```python
from build123d import *

# Parameters (mm, degrees)
BOSS_EXTRUDE1_DEPTH     = 10
SKETCH2_W               = 17.2
SKETCH2_H               = 43
CUT_EXTRUDE1_DEPTH      = 72.414284285
SKETCH3_W               = 90
SKETCH3_H               = 34
SKETCH3_W_2             = 80
SKETCH3_H_2             = 24
BOSS_EXTRUDE3_DEPTH     = 15
SKETCH4_W               = 49.6
SKETCH4_H               = 5
BOSS_EXTRUDE4_DEPTH     = 10
SKETCH5_W               = 15
SKETCH5_H               = 22
BOSS_EXTRUDE5_DEPTH     = 5
SKETCH6_W               = 90
SKETCH6_H               = 77
BOSS_EXTRUDE6_DEPTH     = 15
BOSS_EXTRUDE8_DEPTH     = 39
CHAMFER1_SIZE           = 64
CHAMFER1_SIZE_2         = 3.354097874
CHAMFER2_SIZE           = 64
CHAMFER2_SIZE_2         = 11.405813635
CHAMFER3_SIZE           = 64
CHAMFER3_SIZE_2         = 13.775745352
CUT_EXTRUDE3_DEPTH      = 95.500525601
CUT_EXTRUDE3_DEPTH_BACK = 95.500525601
SKETCH10_W              = 50
SKETCH10_H              = 27
SKETCH15_R              = 8
CUT_EXTRUDE5_DEPTH      = 122.227059686
CUT_EXTRUDE6_DEPTH      = 2.5
SKETCH18_W              = 29.6
SKETCH18_H              = 43
CUT_EXTRUDE7_DEPTH      = 10
CUT_EXTRUDE8_DEPTH      = 15
SKETCH21_W              = 29.6
SKETCH21_H              = 33
BOSS_EXTRUDE10_DEPTH    = 2.5
SKETCH23_W              = 2.05
SKETCH23_H              = 13
BOSS_EXTRUDE11_DEPTH    = 15
SKETCH24_W              = 90
SKETCH24_H              = 72
CUT_EXTRUDE9_DEPTH      = 54


with BuildPart() as part:
    # Sketch1 → Boss-Extrude1 (new body)
    with BuildSketch(Plane(origin=(0, 0, 0), x_dir=(1, 0, 0), z_dir=(0, 1, 0))):
        with BuildLine():
            Line((-35, 50), (35, 50))
            ThreePointArc((35, 50), (45.606601718, 45.606601718), (50, 35))
            Line((50, 35), (50, -35))
            ThreePointArc((50, -35), (45.606601718, -45.606601718), (35, -50))
            Line((35, -50), (-35, -50))
            ThreePointArc((-35, -50), (-45.606601718, -45.606601718), (-50, -35))
            Line((-50, -35), (-50, 35))
            ThreePointArc((-50, 35), (-45.606601718, 45.606601718), (-35, 50))
        make_face()
    extrude(amount=BOSS_EXTRUDE1_DEPTH)

    # Sketch2 → Cut-Extrude1 (cut, through all)
    with BuildSketch(Plane(origin=(0, 10, 0), x_dir=(1, 0, 0), z_dir=(0, 1, 0))):
        with Locations((-33.4, 18.5)):
            Rectangle(SKETCH2_W, SKETCH2_H)
        with Locations((33.4, 18.5)):
            Rectangle(SKETCH2_W, SKETCH2_H)
    extrude(amount=-CUT_EXTRUDE1_DEPTH, mode=Mode.SUBTRACT)

    # Sketch3 → Boss-Extrude3 (add)
    with BuildSketch(Plane(origin=(0, 10, 0), x_dir=(1, 0, 0), z_dir=(0, 1, 0))):
        with Locations((0, -20)):
            Rectangle(SKETCH3_W, SKETCH3_H)
        with Locations((0, -20)):
            Rectangle(SKETCH3_W_2, SKETCH3_H_2, mode=Mode.SUBTRACT)
    extrude(amount=BOSS_EXTRUDE3_DEPTH)

    # Sketch4 → Boss-Extrude4 (add)
    with BuildSketch(Plane(origin=(0, 10, 0), x_dir=(1, 0, 0), z_dir=(0, 1, 0))):
        with Locations((0, 10)):
            Rectangle(SKETCH4_W, SKETCH4_H)
        with Locations((0, 27)):
            Rectangle(SKETCH4_W, SKETCH4_H)
    extrude(amount=BOSS_EXTRUDE4_DEPTH)

    # Sketch5 → Boss-Extrude5 (add)
    with BuildSketch(Plane(origin=(0, 20, 0), x_dir=(1, 0, 0), z_dir=(0, 1, 0))):
        with Locations((-17.3, 18.5)):
            Rectangle(SKETCH5_W, SKETCH5_H)
        with Locations((17.3, 18.5)):
            Rectangle(SKETCH5_W, SKETCH5_H)
    extrude(amount=BOSS_EXTRUDE5_DEPTH)

    # Sketch6 → Boss-Extrude6 (add)
    with BuildSketch(Plane(origin=(0, 10, 0), x_dir=(1, 0, 0), z_dir=(0, 1, 0))):
        with BuildLine():
            Line((-50, 35), (-50, -35))
            ThreePointArc((-50, -35), (-45.606601718, -45.606601718), (-35, -50))
            Line((-35, -50), (35, -50))
            ThreePointArc((35, -50), (45.606601718, -45.606601718), (50, -35))
            Line((50, -35), (50, 35))
            ThreePointArc((50, 35), (45.606601718, 45.606601718), (35, 50))
            Line((35, 50), (-35, 50))
            ThreePointArc((-35, 50), (-45.606601718, 45.606601718), (-50, 35))
        make_face()
        with Locations((0, 1.5)):
            Rectangle(SKETCH6_W, SKETCH6_H, mode=Mode.SUBTRACT)
    extrude(amount=BOSS_EXTRUDE6_DEPTH)

    # Sketch9 → Boss-Extrude8 (add)
    with BuildSketch(Plane(origin=(0, 25, 0), x_dir=(1, 0, 0), z_dir=(0, 1, 0))):
        with BuildLine():
            Line((-50, 35), (-50, -35))
            ThreePointArc((-50, -35), (-45.606601718, -45.606601718), (-35, -50))
            Line((-35, -50), (35, -50))
            ThreePointArc((35, -50), (45.606601718, -45.606601718), (50, -35))
            Line((50, -35), (50, 35))
            ThreePointArc((50, 35), (45.606601718, 45.606601718), (35, 50))
            Line((35, 50), (-35, 50))
            ThreePointArc((-35, 50), (-45.606601718, 45.606601718), (-50, 35))
        make_face()
        with BuildLine():
            Line((-45, 35), (-45, -32))
            Line((-45, -32), (45, -32))
            Line((45, -32), (45, 35))
            ThreePointArc((45, 35), (44.659258263, 37.588190451), (43.660254038, 40))
            Line((43.660254038, 40), (-43.660254038, 40))
            ThreePointArc((-43.660254038, 40), (-44.659258263, 37.588190451), (-45, 35))
        make_face(mode=Mode.SUBTRACT)
    extrude(amount=BOSS_EXTRUDE8_DEPTH)

    # Chamfer1
    # the kernel refuses this chamfer: 64, 3.354097874 mm, written as the material it takes off along each edge
    with BuildSketch(Plane(origin=(-35, 64, 50), x_dir=(0, -0.9999979738662979, 0.002013023422382214), z_dir=(1, 0, 0)), Plane(origin=(50, 64, 35), x_dir=(0.002013023422382214, -0.9999979738662979, 0), z_dir=(0, 0, -1)), Plane(origin=(-50, 64, -35), x_dir=(-0.002013023422382214, -0.9999979738662979, 0), z_dir=(0, 0, 1)), Plane(origin=(35, 64, -50), x_dir=(0, -0.9999979738662979, -0.002013023422382214), z_dir=(-1, 0, 0))) as chamfer1_piece_1:
        Polygon((CHAMFER1_SIZE * 0.999997973866, CHAMFER1_SIZE * 0.00201302342238), (-CHAMFER1_SIZE_2 * 0.00201302342245, CHAMFER1_SIZE_2 * 0.9999979739), (0, 0), align=None)
    extrude(amount=70, mode=Mode.SUBTRACT)
    with BuildSketch(Plane(origin=(35, 64, 35), x_dir=(0, 0, 1), z_dir=(-1, 0, 0))) as chamfer1_piece_2:
        Polygon((15, -CHAMFER1_SIZE), (15 - CHAMFER1_SIZE_2, 0), (15, 0), align=None)
    revolve(axis=Axis((35, 64, 35), (0, 1, 0)), revolution_arc=90, mode=Mode.SUBTRACT)
    with BuildSketch(Plane(origin=(-35, 64, 35), x_dir=(-1, 0, 0), z_dir=(0, 0, -1))) as chamfer1_piece_3:
        Polygon((15, -CHAMFER1_SIZE), (15 - CHAMFER1_SIZE_2, 0), (15, 0), align=None)
    revolve(axis=Axis((-35, 64, 35), (0, 1, 0)), revolution_arc=90, mode=Mode.SUBTRACT)
    with BuildSketch(Plane(origin=(35, 64, -35), x_dir=(1, 0, 0), z_dir=(0, 0, 1))) as chamfer1_piece_4:
        Polygon((15, -CHAMFER1_SIZE), (15 - CHAMFER1_SIZE_2, 0), (15, 0), align=None)
    revolve(axis=Axis((35, 64, -35), (0, 1, 0)), revolution_arc=90, mode=Mode.SUBTRACT)
    with BuildSketch(Plane(origin=(-35, 64, -35), x_dir=(0, 0, -1), z_dir=(1, 0, 0))) as chamfer1_piece_5:
        Polygon((15 - CHAMFER1_SIZE_2, 0), (15, -CHAMFER1_SIZE), (15, 0), align=None)
    revolve(axis=Axis((-35, 64, -35), (0, 1, 0)), revolution_arc=90, mode=Mode.SUBTRACT)

    # Chamfer2
    # the kernel refuses this chamfer: 64, 11.405813635 mm, written as the material it takes off along each edge
    with BuildSketch(Plane(origin=(201.306482971, 64, -46.645902126), x_dir=(0, -0.9982575003065525, -0.05900816114499234), z_dir=(-1, 0, 0))) as chamfer2_piece_1:
        Polygon((CHAMFER2_SIZE * 0.999977671636, CHAMFER2_SIZE * 0.0066825316561), (-CHAMFER2_SIZE_2 * 0.0590081611462, CHAMFER2_SIZE_2 * 0.998257500326), (0, 0), align=None)
    extrude(amount=402.612965942, mode=Mode.SUBTRACT)

    # Chamfer3
    # the kernel refuses this chamfer: 64, 13.775745352 mm, written as the material it takes off along each edge
    with BuildSketch(Plane(origin=(-201.265469314, 64, 46.645902126), x_dir=(0, -0.9981787050157903, 0.06032638604292662), z_dir=(1, 0, 0))) as chamfer3_piece_1:
        Polygon((CHAMFER3_SIZE * 0.999967974892, CHAMFER3_SIZE * 0.00800307379952), (-CHAMFER3_SIZE_2 * 0.060326386045, CHAMFER3_SIZE_2 * 0.99817870505), (0, 0), align=None)
    extrude(amount=402.530938629, mode=Mode.SUBTRACT)

    # Sketch10 → Cut-Extrude3 (cut, two sides: drawn at the far end of the back side and taken through both)
    with BuildSketch(Plane(origin=(0, 1.307501734, 0), x_dir=(0, 0, 1), z_dir=(-1, 0, 0)).offset(-CUT_EXTRUDE3_DEPTH_BACK)):
        with Locations((-22.129843227, 49.192498266)):
            Rectangle(SKETCH10_W, SKETCH10_H)
    extrude(amount=CUT_EXTRUDE3_DEPTH + CUT_EXTRUDE3_DEPTH_BACK, mode=Mode.SUBTRACT)

    # Sketch15 → Cut-Extrude5 (cut, through all)
    with BuildSketch(Plane.XY.offset(-40)):
        with Locations((-12.75, 20.25)):
            Circle(SKETCH15_R)
        with Locations((12.75, 20.25)):
            Circle(SKETCH15_R)
    extrude(amount=-CUT_EXTRUDE5_DEPTH, mode=Mode.SUBTRACT)

    # Sketch17 → Cut-Extrude6 (cut)
    with BuildSketch(Plane(origin=(0, 0, -29.5), x_dir=(-1, 0, 0), z_dir=(0, 0, -1))):
        Polygon((-24.8, 10), (24.8, 10), (24.8, 25), (9.8, 25), (9.8, 20), (-9.8, 20), (-9.8, 25), (-24.8, 25), align=None)
    extrude(amount=-CUT_EXTRUDE6_DEPTH, mode=Mode.SUBTRACT)

    # Sketch18 → Cut-Extrude7 (cut)
    with BuildSketch(Plane.XZ):
        with Locations((0, -18.5)):
            Rectangle(SKETCH18_W, SKETCH18_H)
    extrude(amount=-CUT_EXTRUDE7_DEPTH, mode=Mode.SUBTRACT)

    # Sketch20 → Cut-Extrude8 (cut)
    with BuildSketch(Plane.XZ.offset(-25)):
        with BuildLine():
            Line((-45, -35), (-45, -40))
            Line((-45, -40), (-43.660254038, -40))
            ThreePointArc((-43.660254038, -40), (-44.659258263, -37.588190451), (-45, -35))
        make_face()
        with BuildLine():
            Line((45, -40), (45, -35))
            ThreePointArc((45, -35), (44.659258263, -37.588190451), (43.660254038, -40))
            Line((43.660254038, -40), (45, -40))
        make_face()
    extrude(amount=-CUT_EXTRUDE8_DEPTH, mode=Mode.SUBTRACT)

    # Sketch21 → Boss-Extrude10 (add)
    with BuildSketch(Plane.XZ):
        with Locations((0, -13.5)):
            Rectangle(SKETCH21_W, SKETCH21_H)
    extrude(amount=-BOSS_EXTRUDE10_DEPTH)

    # Sketch23 → Boss-Extrude11 (add)
    with BuildSketch(Plane(origin=(0, 10, 0), x_dir=(1, 0, 0), z_dir=(0, 1, 0))):
        with Locations((-23.775, 33.5)):
            Rectangle(SKETCH23_W, SKETCH23_H)
        with Locations((23.775, 33.5)):
            Rectangle(SKETCH23_W, SKETCH23_H)
    extrude(amount=BOSS_EXTRUDE11_DEPTH)

    # Sketch24 → Cut-Extrude9 (cut)
    with BuildSketch(Plane(origin=(0, 64, 0), x_dir=(1, 0, 0), z_dir=(0, 1, 0))):
        with Locations((0, 4)):
            Rectangle(SKETCH24_W, SKETCH24_H)
    extrude(amount=-CUT_EXTRUDE9_DEPTH, mode=Mode.SUBTRACT)


solid = part.part
```
Check sheet for the modelled part. Datum: model origin and axes. Units: mm. A direction names the side the tool comes from. Coordinates: 2 decimals unless noted, no trailing zeros. Order: outer loops, then holes, each group sorted by start corner. A loop starts at its lowest first (then second) coordinate and runs counter-clockwise, first axis right, second up. Notation, with made-up numbers: (64.25, 80) -> (85.25, 80) arc R33 cw to (85.25, 119) -> close; hole circle Ø10 at (51.25, 71). An arc over 180 degrees is marked (long way). Write each question's results on one line, items separated by ' | '. Start each with the question number.
1) Section check C-C (x = -12.75). Enter the section's corners in (y, z).
2) Set-up check for faces 4 (the face through (-46, 50, 2.87)), 5 (the face through (-42, 5, -18)), 6 (the face through (11.02, 12.44, -42.74)), 7 (the face through (-1, 10, 11)): record each of +Z, -Z, +X, -X, +Y, -Y from which the full face is reachable in a straight line by a thin tool's end or side.
3) Material ranges on line 1 along X through (y, z) = (20.25, -41.5); line 2 along X through (y, z) = (20.25, -42); line 3 along Z through (x, y) = (-26.5, 36.5), recorded low to high.
4) Draft check along Z on faces 1 (the face through (0, 6, 3)), 2 (the face through (48.72, 24.44, 8.27)), 3 (the face through (0.649, 18.285, -45.794)). Enter one of: pulls with the +Z half, pulls with the -Z half, needs draft (parallel to the pull), parting line crosses it, or undercut.
5) Section check A-A (z = -14). Enter the section's corners in (x, y), and give its area (3 significant figures).
6) Section check B-B (x = -1). Enter the section's corners in (y, z).
7) Section check D-D (y = 20.25). Enter the section's corners in (x, z), and give its area (3 significant figures).
8) Depth check by flat-ended pin: pin 1 (2 mm diameter, centred on y = 27, z = 13.5, fed in from -X); pin 2 (4 mm diameter, centred on x = -1, z = -9.5, fed in from +Y); pin 3 (18.5 mm diameter, centred on x = 12.75, y = 20.25, fed in from +Z). Enter the tip coordinate at first touch or a pass-through.
Checked values:
1) outline: (0, -50) -> (0.09, -50) -> (12.25, -47.19) -> (12.25, -40) -> (0, -40) -> close; (0, -30) -> (2.5, -30) -> (2.5, 3) -> (10, 3) -> (10, 32) -> (64, 32) -> (64, 32.87) -> (0.09, 50) -> (0, 50) -> close; (28.25, -43.49) -> (37, -41.47) -> (37, -40) -> (28.25, -40) -> close
2) face 4: -Z, +X, -X, +Y | face 5: +Y, -Y | face 6: -Z | face 7: +Y
3) line 1: -47.33 to -20.75, -4.75 to 4.75, 20.75 to 47.33 | line 2: -47.05 to -20.75, -4.75 to 4.75, 20.75 to 47.05 | line 3: -41.59 to -40, 32 to 40.24
4) face 1: undercut | face 2: needs draft | face 3: pulls with the -Z half
5) outline: (-50, 0) -> (-42, 0) -> (-42, 10) -> (-45, 10) -> (-45, 37) -> (-48.06, 37) -> close; (-24.8, 0) -> (24.8, 0) -> (24.8, 10) -> (14.8, 10) -> (14.8, 2.5) -> (-14.8, 2.5) -> (-14.8, 10) -> (-24.8, 10) -> close; (42, 0) -> (50, 0) -> (48.06, 37) -> (45, 37) -> (45, 10) -> (42, 10) -> close | area: 632 mm²
6) outline: (0, -50) -> (0.09, -50) -> (37, -41.47) -> (37, -40) -> (0, -40) -> close; (0, -30) -> (2.5, -30) -> (2.5, 3) -> (10, 3) -> (10, 32) -> (64, 32) -> (64, 32.87) -> (0.09, 50) -> (0, 50) -> close
7) outline: (-48.94, -35) arc R13.94 ccw to (-44.35, -45.34) -> (-20.75, -45.34) -> (-20.75, -40) -> (-45, -40) -> (-45, 32) -> (45, 32) -> (45, -40) -> (20.75, -40) -> (20.75, -45.34) -> (44.35, -45.34) arc R13.94 ccw to (48.94, -35) -> (48.94, 35) arc R13.94 ccw to (45.11, 44.59) -> (-45.11, 44.59) arc R13.94 ccw to (-48.94, 35) -> close; (-4.75, -45.34) -> (4.75, -45.34) -> (4.75, -40) -> (-4.75, -40) -> close | area: 2,100 mm²
8) pin 1: x = -48.64 | pin 2: y = 2.5 | pin 3: z = 47.07
